Source: CAD feature listing. Evaluate the final solid. Frame: model axes, mm. Face numbers are marked on the shaded views. A direction names the side the tool comes from. Give positions to 0.01 mm unless a question says otherwise; leave off trailing zeros. Order: outer loops, then holes, each group sorted by start corner. A loop starts at its lowest first (then second) coordinate and runs counter-clockwise, first axis right, second up. Notation, with made-up numbers: (19, -22) -> (74, -22) arc R25 ccw to (74, 17) -> close; hole circle Ø3 at (11, 2.25). An arc over 180 degrees is marked (long way). Answer in a Markdown table with one row per item.
```python
from build123d import *

# Parameters (mm, degrees)
BOSS_EXTRUDE1_DEPTH = 25.4
FILLET4_R           = 7.62
FILLET5_R           = 2.54
FILLET6_R           = 2.54
SKETCH2_R           = 3.2639
CUT_EXTRUDE1_DEPTH  = 10.16
SKETCH3_R           = 4.7625
CUT_EXTRUDE4_DEPTH  = 10.16


with BuildPart() as part:
    # Sketch1 → Boss-Extrude1 (new body)
    with BuildSketch(Plane(origin=(0, 0, 0), x_dir=(0, 0, -1), z_dir=(1, 0, 0))):
        Polygon((-50.8, 0), (50.8, 0), (32.681037195, 11.050662882), (43.390895004, 40.811843798), align=None)
    extrude(amount=BOSS_EXTRUDE1_DEPTH)

    # Fillet4
    fillet4_edges = [part.edges().sort_by_distance(p)[0] for p in [
        (12.7, 11.050662882, -32.681037195),
    ]]
    fillet(fillet4_edges, radius=FILLET4_R)

    # Fillet5
    fillet5_edges = [part.edges().sort_by_distance(p)[0] for p in [
        (12.7, 40.811843798, -43.390895004),
    ]]
    fillet(fillet5_edges, radius=FILLET5_R)

    # Fillet6
    fillet6_edges = [part.edges().sort_by_distance(p)[0] for p in [
        (25.4, 3.906974274, -44.39402035),
        (0, 26.09308805, -38.094203934),
        (25.4, 26.09308805, -38.094203934),
        (0, 11.786560732, -34.769020969),
        (25.4, 11.786560732, -34.769020969),
        (0, 19.238614503, 6.398616724),
        (25.4, 19.238614503, 6.398616724),
        (0, 37.998707408, -40.750789597),
        (25.4, 37.998707408, -40.750789597),
        (0, 3.906974274, -44.39402035),
    ]]
    fillet(fillet6_edges, radius=FILLET6_R)

    # Sketch2 → Cut-Extrude1 (cut)
    with BuildSketch(Plane.XZ):
        with Locations(Location((12.7, 40.64, 0), (0, 0, 270))):
            Circle(SKETCH2_R)
        with Locations(Location((12.7, -40.64, 0), (0, 0, 270))):
            Circle(SKETCH2_R)
    extrude(amount=-CUT_EXTRUDE1_DEPTH, mode=Mode.SUBTRACT)

    # Sketch3 → Cut-Extrude4 (cut)
    with BuildSketch(Plane(origin=(0, 2.54, 0), x_dir=(-1, 0, 0), z_dir=(0, -1, 0))):
        with Locations((-12.7, -40.64)):
            Circle(SKETCH3_R)
        with Locations(Location((-12.7, 40.64, 0), (0, 0, 90))):
            Circle(SKETCH3_R)
    extrude(amount=-CUT_EXTRUDE4_DEPTH, mode=Mode.SUBTRACT)


solid = part.part
```
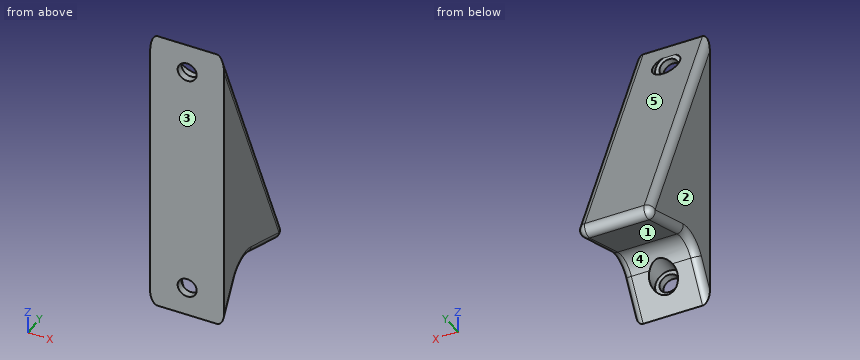
(1) Pull-direction query (Y, two-part tool) for the marked faces 3, 4 and 5; classes: +Y half, -Y half, draft (parallel to the pull), parting line (faces both ways), or undercut.
A:
| item | result |
|---|---|
| face 3 | -Y half |
| face 4 | undercut |
| face 5 | +Y half |
(2) Access query for the marked faces 1 and 2. Directions: +Z, -Z, +X, -X, +Y, -Y. A direction counts if a zero-diameter tool reaches every point of the face in a straight line with its end or side. Return the directions, or none.
A:
| item | result |
|---|---|
| face 1 | -Z, +X, -X |
| face 2 | +Z, -Z, -X, +Y, -Y |
(3) First-contact query: pin 1 Ø4.5 at (x, z) = (11, 39.5) entering from +Y; pin 2 Ø1 at (x, y) = (9.5, 13.5) entering from -Z; pin 3 Ø15 at (x, z) = (12.7, 40.64) entering from +Y; pin 4 Ø5 at (x, z) = (12.7, 40.64) entering from +Y. Flat tips, straight axial feed; report the tip coordinate or a pass-through.
A:
| item | result |
|---|---|
| pin 1 | stops at y = 2.54 |
| pin 2 | stops at z = -34.45 |
| pin 3 | stops at y = 7.65 |
| pin 4 | passes through |
(4) Ray query, probe 1 along X at (y, z) = (1.5, -40.64); probe 2 along Y at (x, z) = (13.75, -44); probe 3 along Z at (x, y) = (22.5, 17). Return the intervals inside material, ascending.
A:
| item | result |
|---|---|
| probe 1 | x = 0 to 9.44, 15.96 to 25.4 |
| probe 2 | y = 0 to 2.54 |
| probe 3 | z = -34.82 to 11.57 |
(5) Section query A-A (x = 12.7). Return the cut outline in (y, z), plus the area to 3 significant figures.
A:
| item | result |
|---|---|
| outline | (0, -50.8) -> (3.29, -45.4) -> (2.54, -45.4) -> (2.54, -43.9) -> (0, -43.9) -> close; (0, -37.38) -> (2.54, -37.38) -> (2.54, -35.88) -> (9.72, -35.88) arc R7.62 cw to (16.9, -34.79) -> (35.29, -41.4) arc R2.54 ccw to (38.48, -38) -> (6.47, 35.88) -> (2.54, 35.88) -> (2.54, 37.38) -> (0, 37.38) -> close; (0, 43.9) -> (2.54, 43.9) -> (2.54, 44.94) -> (0, 50.8) -> close |
| area | 1,660 mm^2 |
